Autodesk Inventor part; units mm, degrees
ref_plane "YZ Plane" through (0, 0, 0) normal (1, 0, 0) x (0, 1, 0)
ref_plane "XZ Plane" through (0, 0, 0) normal (0, 1, 0) x (-1, 0, 0)
ref_plane "XY Plane" through (0, 0, 0) normal (0, 0, 1) x (1, 0, 0)
sketch "Sketch1" plane through (0, 0, 0) normal (0, 1, 0) x (-1, 0, 0)
  line L0 (0, -2.7496) -> (-2.3812, -1.3748)
  line L1 (-2.3812, -1.3748) -> (-2.3813, 1.3748)
  line L2 (-2.3813, 1.3748) -> (0, 2.7496)
  line L3 (0, 2.7496) -> (2.3812, 1.3748)
  line L4 (2.3812, 1.3748) -> (2.3813, -1.3748)
  line L5 (2.3813, -1.3748) -> (0, -2.7496)
  point P0 (0, 0)
  point P1 (0, 0)
  dimension "d0" = 4.7625
extrude "Extrusion1" add sketch "Sketch1" along normal blind 25.4
sketch "Sketch2" plane through (0, 25.4, 0) normal (0, 1, 0) x (1, 0, 0)
  point P0 (0, 0)
  point P1 (0, 0)
hole "Hole1" at (0, 25.4, 0) direction (0, -1, 0) diameter 2.159 end through all
properties part number "standoff"
Model file for the job. Use its own axes, mm. Coordinates: 2 decimals unless noted, no trailing zeros. Order: outer loops, then holes, each group sorted by start corner. A loop starts at its lowest first (then second) coordinate and runs counter-clockwise, first axis right, second up. Notation, with made-up numbers: M -5,66.5 L 27,66.5 A8 cw 27,80.5 Z; hole C 73,16 d2. An arc over 180 degrees is marked long. Answer as CSV lines item,"result".
(1) Wall check: line 1 along X through (y, z) = (11.5, 0); line 2 along Z through (x, y) = (0.15, 18.75); line 3 along X through (y, z) = (23.5, 0.9). Give the ranges that are in metal, low to high.
Geometry says:
line 1,"x = -2.38 to -1.08, 1.08 to 2.38"
line 2,"z = -2.66 to -1.07, 1.07 to 2.66"
line 3,"x = -2.38 to -0.6, 0.6 to 2.38"
(2) Band-saw the part on A-A, the plane y = 12.5. List the corners of the cut face in (x, z).
Geometry says:
outline,"M -2.38,-1.37 L 0,-2.75 L 2.38,-1.37 L 2.38,1.37 L 0,2.75 L -2.38,1.37 Z; hole C 0,0 d2.16"
(3) Band-saw the part on B-B, the plane z = 0. List the corners of the cut face in (x, y), then the cut area to 3 significant figures.
Geometry says:
outline,"M -2.38,0 L -1.08,0 L -1.08,25.4 L -2.38,25.4 Z; M 1.08,0 L 2.38,0 L 2.38,25.4 L 1.08,25.4 Z"
area,"66.1 mm2"
(4) Band-saw the part on C-C, the plane x = 0.75. List the corners of the cut face in (y, z).
Geometry says:
outline,"M 0,-2.32 L 25.4,-2.32 L 25.4,-0.78 L 0,-0.78 Z; M 0,0.78 L 25.4,0.78 L 25.4,2.32 L 0,2.32 Z"
(5) Flat gauge pins, fed straight in: pin 1 (2 mm diameter, centred on x = -1.5, y = 18, fed in from -Z); pin 2 (1.7 mm diameter, centred on x = 0, z = 0, fed in from +Y); pin 3 (1 mm diameter, centred on x = 1, y = 12, fed in from +Z); pin 4 (1 mm diameter, centred on y = 6.5, z = -2, fed in from +X). Where does each tip first touch, or does it go through?
Geometry says:
pin 1,"stops at z = -2.46"
pin 2,"passes through"
pin 3,"stops at z = 2.46"
pin 4,"stops at x = 2.16"
(6) Band-saw the part on D-D, the plane z = 1.65. List the corners of the cut face in (x, y), then the cut area to 3 significant figures.
Geometry says:
outline,"M -1.9,0 L 1.9,0 L 1.9,25.4 L -1.9,25.4 Z"
area,"96.8 mm2"
